Here's how the part is built. I have some questions about the finished solid (model axes, mm). Give positions to 0.01 mm unless a question says otherwise; leave off trailing zeros. Write each loop counter-clockwise with the first axis right and the second up, starting at its lowest first coordinate (ties: lowest second). Pieces come first, ordered by that corner, then holes. Notation, with made-up numbers: M -7.5,21 L 47.5,21 A25 cw 47.5,43 Z; hole C 65.5,13.5 d8. An arc over 180 degrees is marked long. Answer as CSV lines item,"result". Start each with the question number.
Q1. Suppose I cut it at A-A (x = 10). Write out the boundary of the cut face in (y, z).
Q2. Suppose I cut it at D-D (y = 13). Write out the boundary of the cut face in (x, z).
Q3. Thinking about a two-plate mould opening in X: for faces 1 (the flat face through (-11.4, -1.1, 0)), 2 (the cylindrical face through (-2.38, -10.74, -3.6)), 3 (the flat face through (9.238, -17.295, -3.599)), which applies, +X half, -X half, draft (parallel to the pull), parting line (faces both ways), or undercut?
Q4. For pin 1 (1.5 mm diameter, centred on y = -8.5, z = -2, fed in from +X); pin 2 (3 mm diameter, centred on x = -7, z = -5.5, fed in from -Y); pin 3 (4 mm diameter, centred on x = 2.5, z = -5.5, fed in from -Y), each with a flat end and sliding along its axis, tell me the tip position at first contact or that it passes through.
Q5. Suppose I cut it at C-C (z = -1). Write out the boundary of the cut face in (x, y), then the cut area to 3 significant figures.
Q6. Suppose I cut it at B-B (y = 2.5). Write out the boundary of the cut face in (x, z).
Q7. If I drill on line 1 along X through (y, z) = (-6, -5.25); line 2 along Y through (x, z) = (0, -4); line 3 along X through (y, z) = (1.5, -7), over which ranges is the centre line in solid material (lowest first)?
```python
from build123d import *

# Parameters (mm, degrees)
F2_DEPTH = 7
F3_DEPTH = 2.6
F0_R     = 11
F4_DEPTH = 25
F5_DEPTH = 2.3


with BuildPart() as f2:
    # F1 (on Top) → F2 (new body)
    with BuildSketch(Plane.XY):
        Polygon((-23.813827268, -4.4963938878), (-3.0825526201, -24.0377577259), (21.9087049767, -10.3597574001), (16.6228769451, 17.6350755374), (-11.6352020338, 21.2588334764), align=None)
    extrude(amount=-F2_DEPTH)

    # F3 (add): a face of the model
    f3_faces = [f2.faces().sort_by_distance(p)[0] for p in [
        (0, 0, -7),
    ]]
    extrude(f3_faces, amount=F3_DEPTH)

    # F0 (on Top) → F4 (cut)
    with BuildSketch(Plane.XY):
        Circle(F0_R)
    extrude(amount=-F4_DEPTH, mode=Mode.SUBTRACT)

    # F5 (cut): a face of the model
    f5_faces = [f2.faces().sort_by_distance(p)[0] for p in [
        (-13.0067285738, -13.7987330141, -9.6),
    ]]
    extrude(f5_faces, amount=-F5_DEPTH, mode=Mode.SUBTRACT)


solid = f2.part
```
Resolved:
1,outline,"M -16.88,-7.3 L -4.58,-7.3 L -4.58,0 L -16.88,0 Z; M 4.58,-7.3 L 18.48,-7.3 L 18.48,0 L 4.58,0 Z"
2,outline,"M -15.54,-7.3 L 17.5,-7.3 L 17.5,0 L -15.54,0 Z"
3,face 1,"draft"
3,face 2,"undercut"
3,face 3,"+X half"
4,pin 1,"x = 21.7"
4,pin 2,"y = -21.76"
4,pin 3,"y = -22.08"
5,outline,"M -23.81,-4.5 L -3.08,-24.04 L 21.91,-10.36 L 16.62,17.64 L -11.64,21.26 Z; hole C 0,0 d22"
5,area,"1,020 mm^2"
6,outline,"M -20.51,-7.3 L -10.71,-7.3 L -10.71,0 L -20.51,0 Z; M 10.71,-7.3 L 19.48,-7.3 L 19.48,0 L 10.71,0 Z"
7,line 1,"-22.22 to -9.22, 9.22 to 21.09"
7,line 2,"-22.35 to -11, 11 to 19.77"
7,line 3,"-20.98 to -10.9, 10.9 to 19.67"
